Answer from the drawing. Dimensions are ordinates in mm from the lowest x, y and z of the part. A direction names the side the tool comes from. Give positions to 0.01 mm unless a question says otherwise; leave off trailing zeros. Loops run counter-clockwise (first coordinate to the right, second up) from the corner with the lowest first, then second, coordinate; pieces in that order, holes last.
Item 1: A tool of negligible diameter and unlimited length cuts with its end or side. For the marked faces 1, 2 and 3, from which of +Z, -Z, +X, -X, +Y, -Y can it reach the whole face along a straight path? Write none if from no direction.
Item 2: Consider line 1 along Y through (x, z) = (19, 8.5); line 2 along Y through (x, z) = (28.5, 1.55); line 3 along Z through (x, y) = (25, 18.5). Determine where each line is inside the solid, lowest interval first.
Item 3: Section A-A, the plane y = 31.5 is taken. Give the vertices of the cut face in (x, z).
Item 4: Section C-C, the plane z = 18 is taken. Give the vertices of the cut face in (x, y).
Item 5: Section B-B, the plane x = 7.5 is taken. Give the vertices of the cut face in (y, z), and give its area (3 significant figures).
Item 6: The mould has two halves that part along X. Classify the marked faces 4, 5, 6 and 7: pulls with the +X half, pulls with the -X half, needs draft (parallel to the pull), parting line crosses it, or undercut.
Item 7: Each of these flat-tipped pins is pushed along its axis until it touches: pin 1 Ø4 at (x, y) = (7.5, 11.5) entering from +Z; pin 2 Ø4.5 at (y, z) = (10, 12) entering from -X; pin 3 Ø6 at (x, y) = (11, 4.5) entering from -Z; pin 4 Ø5 at (x, z) = (8, 7) entering from +Y. Where does it stop, or does it pass through?
Item 8: Section D-D, the plane y = 11.5 is taken. Give the vertices of the cut face in (x, z), and give its area (3 significant figures).
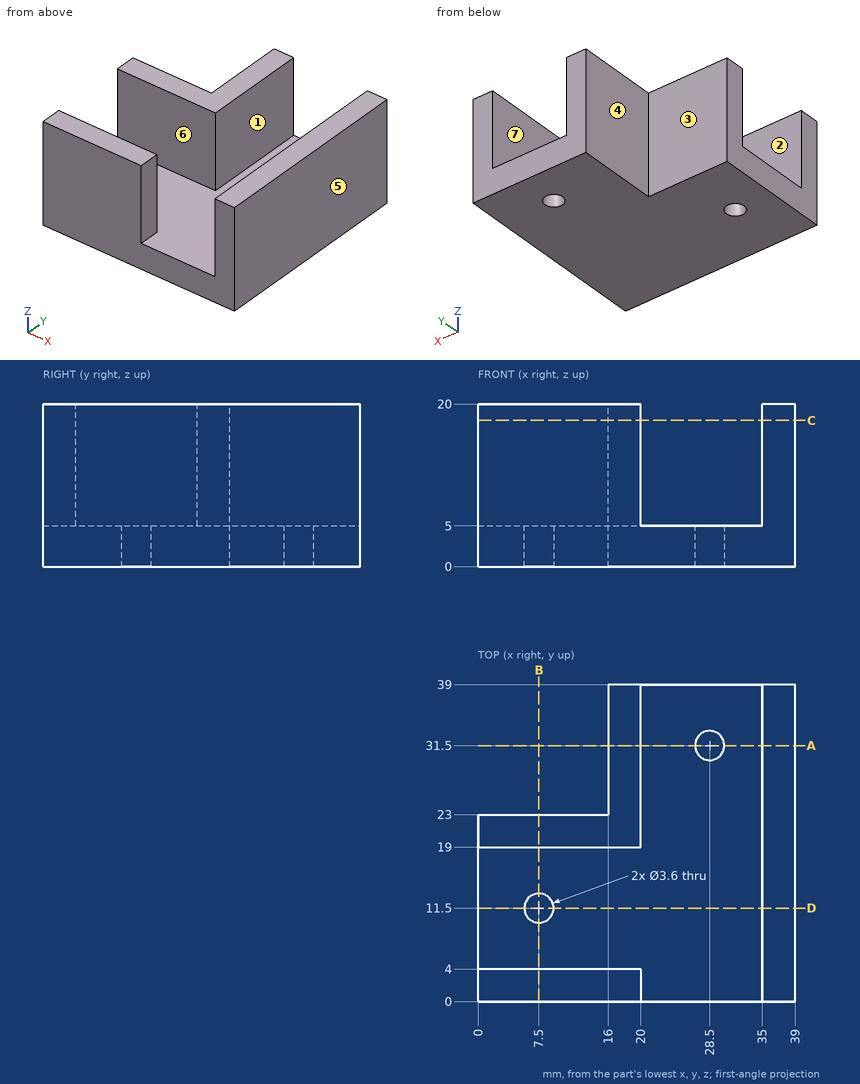
Worked answers:
1. face 1: +Z, +Y, -Y
1. face 2: +Z, -X
1. face 3: +Z, -Z, -X, +Y
2. line 1: y = 0 to 4, 19 to 39
2. line 2: y = 0 to 29.7, 33.3 to 39
2. line 3: z = 0 to 5
3. outline: (16, 0) - (26.7, 0) - (26.7, 5) - (20, 5) - (20, 20) - (16, 20) - close; (30.3, 0) - (39, 0) - (39, 20) - (35, 20) - (35, 5) - (30.3, 5) - close
4. outline: (0, 0) - (20, 0) - (20, 4) - (0, 4) - close; (0, 19) - (20, 19) - (20, 39) - (16, 39) - (16, 23) - (0, 23) - close; (35, 0) - (39, 0) - (39, 39) - (35, 39) - close
5. outline: (0, 0) - (9.7, 0) - (9.7, 5) - (4, 5) - (4, 20) - (0, 20) - close; (13.3, 0) - (23, 0) - (23, 20) - (19, 20) - (19, 5) - (13.3, 5) - close
5. area: 217 mm2
6. face 4: pulls with the -X half
6. face 5: pulls with the +X half
6. face 6: needs draft
6. face 7: undercut
7. pin 1: stops at z = 5
7. pin 2: stops at x = 35
7. pin 3: stops at z = 0
7. pin 4: stops at y = 23
8. outline: (0, 0) - (5.7, 0) - (5.7, 5) - (0, 5) - close; (9.3, 0) - (39, 0) - (39, 20) - (35, 20) - (35, 5) - (9.3, 5) - close
8. area: 237 mm2
